Can you work these out from the model? Positions are in its coordinate system, mm. A direction names the side the tool comes from. Give positions to 0.01 mm unless a question says otherwise; leave off trailing zeros. Order: outer loops, then holes, each group sorted by start corner. A loop starts at its lowest first (then second) coordinate and runs counter-clockwise, first axis right, second up. Notation, with made-up numbers: M 25.25,25 L 67.25,25 A27 ccw 67.25,44 Z; hole C -23.75,-12 d11. An arc over 180 degrees is marked long. Write each question's results on one line, items separated by ' | '.
Autodesk Inventor part; units mm, degrees
ref_plane "Work Plane1" through (0, 0, 31) normal (0, 0, -1) x (-1, 0, 0)
ref_plane "YZ Plane" through (0, 0, 0) normal (1, 0, 0) x (0, 1, 0)
ref_plane "XZ Plane" through (0, 0, 0) normal (0, 1, 0) x (-1, 0, 0)
sketch "Sketch1" plane through (0, 0, 0) normal (0, 0, 1) x (1, 0, 0)
  line L0 (11.1109, 10.667) -> (-10.8891, 10.667)
  arc A0 (17.1109, 4.667) -> (11.1109, 10.667) centre (11.1109, 4.667) ccw
  arc A1 (-10.8891, 10.667) -> (-16.8891, 4.667) centre (-10.8891, 4.667) ccw
  line L1 (17.1109, -11.333) -> (17.1109, 4.667)
  arc A2 (17.1109, 4.667) -> (11.1109, 10.667) centre (11.1109, 4.667) ccw
  line L2 (11.1109, 10.667) -> (-10.8891, 10.667)
  arc A3 (-10.8891, 10.667) -> (-16.8891, 4.667) centre (-10.8891, 4.667) ccw
  line L3 (-16.8891, 4.667) -> (-16.8891, -11.333)
  line L4 (16.1109, 4.667) -> (16.1109, -11.333)
  line L5 (17.1109, -11.333) -> (-16.8891, -11.333)
  line L6 (-15.8891, -11.333) -> (-15.8891, 4.667)
  arc A4 (-10.8891, 9.667) -> (-15.8891, 4.667) centre (-10.8891, 4.667) ccw
  line L7 (-10.8891, 9.667) -> (11.1109, 9.667)
  arc A5 (16.1109, 4.667) -> (11.1109, 9.667) centre (11.1109, 4.667) ccw
  line L8 (-16.8891, -3.333) -> (17.1109, -3.333)
  line L9 (-15.8891, -3.333) -> (-15.8891, 7.1792)
  line L10 (-15.8891, 2.667) -> (-13.8891, 2.667)
  line L11 (16.1109, -3.333) -> (-15.8891, -3.333)
  circle A6 centre (-13.8891, 2.667) radius 2
  line L12 (20.9541, 5.1792) -> (19.218, 5.1792)
  circle A7 centre (-13.8891, 2.667) radius 1.6
  line L13 (-13.8891, 4.267) -> (-15.8891, 4.267)
  line L14 (-15.8891, 4.267) -> (-15.8891, 1.067)
  line L15 (-15.8891, 1.067) -> (-13.8891, 1.067)
  line L16 (-13.8891, 1.067) -> (-13.8891, 4.267)
  circle A8 centre (13.4109, 2.667) radius 2
  circle A9 centre (13.4109, 2.667) radius 1.6
  line L17 (16.1109, 4.667) -> (16.1109, -3.333)
  line L18 (13.4109, 4.267) -> (16.1109, 4.267)
  line L19 (16.1109, 4.267) -> (16.1109, 1.267)
  line L20 (16.1109, 1.267) -> (13.4109, 1.267)
  line L21 (13.4109, 1.267) -> (13.4109, 4.267)
  point P0 (0, 0)
  point P1 (16.1109, -3.333)
  point P2 (-15.8891, -3.333)
  point P3 (17.1109, 4.667)
  point P4 (-16.8891, 4.667)
  point P5 (-13.8891, 2.667)
  point P6 (-15.8891, 1.067)
  point P7 (-15.0891, 1.067)
  point P8 (-15.0891, 4.267)
  point P9 (-15.8891, 4.267)
  point P10 (14.8392, 1.267)
  point P11 (16.1109, 1.267)
  point P12 (16.1109, 4.267)
  point P13 (14.6109, 4.267)
  dimension "d16" = 3.2
  dimension "d18" = 3.2
  dimension "d19" = 27.3
  dimension "d0" = 1
  dimension "d3" = 22
  dimension "d4" = 34
  dimension "d5" = 16
  dimension "d6" = 6
  dimension "d7" = 5
  dimension "d8" = 9.667
  dimension "d9" = 10.667
  dimension "d10" = 11.333
  dimension "d11" = 8
  dimension "d12" = 22
  dimension "d13" = 34
  dimension "d14" = 6
  dimension "d15" = 4
  dimension "d17" = 4
  dimension "d20" = 0
  dimension "d21" = 0
extrude "Extrusion1" add sketch "Sketch1" along normal blind 31 contours A0 L1 L8 L4 A5 L7 A4 L6 L3 A1 L0 | L1 L5 L4 L8 | L8 L6 L5 L3 | L4 L5 L6 L8
extrude "Extrusion2" add sketch "Sketch1" along normal blind 5 contours L20 A8 L18 L4 | L6 A6 L15 | L20 A9 L18 A8 | A8 L18 A9 L20 | A6 L13 A7 L10 | L6 L13 A6 | L10 A7 L15 A6 | L15 A7 L13 A6
ref_plane "Work Plane1" through (0, 0, 31) normal (0, 0, -1) x (-1, 0, 0)
sketch "Sketch2" plane through (0, 0, 31) normal (0, 0, 1) x (1, 0, 0)
  line L0 (-15.8891, -3.333) -> (-15.8891, 1.067)
  line L1 (-15.8891, -3.333) -> (-15.8891, 5)
  line L2 (16.1109, -3.333) -> (-15.8891, -3.333)
  line L3 (-15.8891, -3.333) -> (16.1109, -3.333)
  line L4 (16.1109, -3.333) -> (16.1109, 4.667)
  arc A0 (16.1109, 4.667) -> (11.1109, 9.667) centre (11.1109, 4.667) ccw
  circle A1 centre (11.1109, 4.667) radius 5
  circle A2 centre (-10.8708, 4.667) radius 5
  line L5 (-10.8708, 10.6741) -> (11.1109, 10.6741)
  line L6 (-10.8708, 9.667) -> (11.1109, 9.667)
  line L7 (-10.8708, 9.667) -> (11.1109, 9.667)
  line L8 (-15.8891, -3.333) -> (16.1109, -3.333)
  line L9 (16.1109, 4.667) -> (16.1109, -3.333)
  line L10 (-15.8891, -3.333) -> (-15.8708, 4.6784)
  point P0 (0, 0)
  dimension "d25" = 10
extrude "Extrusion3" add sketch "Sketch2" against normal blind 1
properties part number "SERVO.housing_3DPrint"
(1) Will these pins go through, and if not, where does the flat tip stop? P1, Ø0.6, axis at x = -15.5, z = 2.5, coming from the +Y side; P2, Ø1.6, axis at x = 15, z = 2.5, coming from the +Y side.
Data:
P1: stops at y = 8.84 | P2: stops at y = 9.81
(2) Imagine slicing it at D-D, the plane y = -2.75. Write out the boundary of the cut face in (x, z), plus the area to 3 significant figures.
Data:
outline: M -16.89,0 L -15.89,0 L -15.89,31 L -16.89,31 Z; M -15.89,30 L 16.11,30 L 16.11,0 L 17.11,0 L 17.11,31 L -15.89,31 Z | area: 94.0 mm2
(3) We'd pull the mould along Y, two halves only. Please class faces 4 (the face through (0, -11.333, 15)), 5 (the face through (0, -6, 0)), 6 (the face through (13.06, 4.23, 2.46)): +Y half, -Y half, draft (parallel to the pull), parting line (faces both ways), or undercut.
Data:
face 4: -Y half | face 5: draft | face 6: undercut
(4) Imagine slicing it at B-B, the plane x = -4.5. Write out the boundary of the cut face in (y, z).
Data:
outline: M -11.33,0 L -3.33,0 L -3.33,30 L 9.67,30 L 9.67,0 L 10.67,0 L 10.67,31 L -11.33,31 Z
(5) I need wall thicknesses on L1, parallel to Y at x = -9.5, z = 23.5; L2, parallel to X at y = 2.5, z = 29.5; L3, parallel to Z at x = -13, y = -0.75. Which ranges of each line are inside material? Lowest first, please. Write a range as from..to.
Data:
L1: y = -11.33..-3.33, 9.67..10.67 | L2: x = -16.89..-15.89, 16.11..17.11 | L3: z = 30..31
(6) Imagine slicing it at C-C, the plane z = 21. Write out the boundary of the cut face in (x, y).
Data:
outline: M -16.89,-11.33 L 17.11,-11.33 L 17.11,4.67 A6 ccw 11.11,10.67 L -10.89,10.67 A6 ccw -16.89,4.67 Z; hole M -15.89,-3.33 L 16.11,-3.33 L 16.11,4.67 A5 ccw 11.11,9.67 L -10.89,9.67 A5 ccw -15.89,4.67 Z
(7) For faces 1 (the face through (-12.41, 3.28, 2.46)), 2 (the face through (0, 0, 31)), 3 (the face through (-15.889, 1, 15)), which set-ups out of +Z, -Z, +X, -X, +Y, -Y let a thin tool reach every point of the face, with its end or its side?
Data:
face 1: -Z | face 2: +Z, +X, -X, +Y, -Y | face 3: none
(8) Imagine slicing it at A-A, the plane y = 9. Write out the boundary of the cut face in (x, z).
Data:
outline: M -15.04,0 L -13.38,0 L -13.38,31 L -15.04,31 Z; M -13.37,30 L 13.61,30 L 13.61,0 L 15.26,0 L 15.26,31 L -13.37,31 Z
